Autodesk Inventor part; units mm, degrees
ref_plane "Piano di lavoro9" through (123.3139, -0.0528, 92.5382) normal (1, 0, 0) x (0, 0, -1)
ref_plane "Piano di lavoro11" through (123.3139, -0.0528, 92.5382) normal (1, 0, 0) x (0, 0, -1)
ref_plane "YZ Plane" through (0, 0, 0) normal (1, 0, 0) x (0, 1, 0)
ref_plane "Piano di lavoro9" through (123.3139, -0.0528, 92.5382) normal (1, 0, 0) x (0, 0, -1)
sketch "Schizzo5" plane through (123.3139, -0.0528, 92.5382) normal (1, 0, 0) x (0, 0, -1)
  line L0 (71.3231, 66.1847) -> (134.8231, 66.1847)
  line L1 (134.8231, 66.1847) -> (134.8231, 34.6847)
  line L2 (134.8231, 34.6847) -> (71.3231, 34.6847)
  line L3 (71.3231, 34.6847) -> (71.3231, 66.1847)
  line L4 (71.3231, 34.6847) -> (81.3231, 34.6847)
  line L5 (81.3231, 34.6847) -> (81.3231, 29.6847)
  line L6 (81.3231, 29.6847) -> (71.3231, 29.6847)
  line L7 (134.8231, 34.6847) -> (124.8231, 34.6847)
  line L8 (124.8231, 34.6847) -> (124.8231, 29.6847)
  line L9 (124.8231, 29.6847) -> (134.8231, 29.6847)
  line L10 (71.3231, 66.1847) -> (81.3231, 66.1847)
  line L11 (81.3231, 66.1847) -> (81.3231, 69.1847)
  line L12 (81.3231, 69.1847) -> (71.3231, 69.1847)
  line L13 (134.8231, 66.1847) -> (124.8231, 66.1847)
  line L14 (124.8231, 66.1847) -> (124.8231, 69.1847)
  line L15 (124.8231, 69.1847) -> (134.8231, 69.1847)
  line L16 (71.3231, 69.1847) -> (68.3231, 69.1847)
  line L17 (68.3231, 69.1847) -> (68.3231, 29.6847)
  line L18 (68.3231, 29.6847) -> (71.3231, 29.6847)
  line L19 (71.3231, 34.6847) -> (71.3231, 66.1847)
  line L20 (134.8231, 69.1847) -> (137.8231, 69.1847)
  line L21 (137.8231, 69.1847) -> (137.8231, 29.6847)
  line L22 (137.8231, 29.6847) -> (134.8231, 29.6847)
  point P0 (92.5382, 0.0528)
  dimension "d18" = 63.5
  dimension "d19" = 31.5
  dimension "d20" = 10
  dimension "d21" = 5
  dimension "d22" = 10
  dimension "d23" = 5
  dimension "d24" = 10
  dimension "d25" = 3
  dimension "d26" = 10
  dimension "d27" = 3
  dimension "d28" = 3
  dimension "d29" = 3
extrude "Estrusione3" add sketch "Schizzo5" against normal blind 100 contours L3 L2 L5 L6 L18 L17 L16 L12 L11 L0 | L14 L15 L20 L21 L22 L9 L8 L2 L1 L0
ref_plane "Piano di lavoro11" through (123.3139, -0.0528, 92.5382) normal (1, 0, 0) x (0, 0, -1)
sketch "Schizzo6" plane through (123.3139, -0.0528, 92.5382) normal (1, 0, 0) x (0, 0, -1)
  line L0 (71.3231, 66.1847) -> (81.3231, 66.1847)
  line L1 (81.3231, 34.6847) -> (71.3231, 34.6847)
  line L2 (81.3231, 29.6847) -> (81.3231, 34.6847)
  line L3 (134.8231, 66.1847) -> (134.8231, 34.6847)
  line L4 (71.3231, 34.6847) -> (71.3231, 66.1847)
  line L5 (68.3231, 99.6847) -> (137.155, 99.6847)
  line L6 (124.8231, 69.1847) -> (137.8231, 69.1847)
  line L7 (137.8231, 69.1847) -> (134.8231, 69.1847)
  line L8 (134.8231, 69.1847) -> (134.8231, 79.6847)
  line L9 (137.8231, 79.6847) -> (137.8231, 69.1847)
  line L10 (71.3231, 69.1847) -> (71.3231, 79.6847)
  line L11 (68.3231, 79.6847) -> (68.3231, 69.1847)
  line L12 (115.0731, 79.6847) -> (134.8231, 79.6847)
  line L13 (137.8231, 79.6847) -> (137.8231, 82.6847)
  line L14 (137.8231, 82.6847) -> (118.0731, 82.6847)
  line L15 (91.0731, 79.6847) -> (71.3231, 79.6847)
  line L16 (68.3231, 79.6847) -> (68.3231, 82.6847)
  line L17 (68.3231, 82.6847) -> (88.0731, 82.6847)
  line L18 (91.0731, 82.6847) -> (93.0731, 82.6847)
  line L19 (93.0731, 82.6847) -> (93.0731, 79.6847)
  line L20 (93.0731, 79.6847) -> (91.0731, 79.6847)
  line L21 (115.0731, 82.6847) -> (113.0731, 82.6847)
  line L22 (113.0731, 82.6847) -> (113.0731, 79.6847)
  line L23 (113.0731, 79.6847) -> (115.0731, 79.6847)
  line L24 (91.0731, 82.6847) -> (91.0731, 84.6847)
  line L25 (88.0731, 82.6847) -> (88.0731, 85.6847)
  line L26 (93.0731, 85.6847) -> (93.0731, 84.6847)
  line L27 (93.0731, 84.6847) -> (91.0731, 84.6847)
  line L28 (113.0731, 84.6847) -> (115.0731, 84.6847)
  line L29 (93.0731, 85.6847) -> (93.0731, 86.6847)
  line L30 (88.0731, 85.6847) -> (88.0731, 86.6847)
  line L31 (88.0731, 86.6847) -> (93.0731, 86.6847)
  line L32 (113.0731, 84.6847) -> (113.0731, 86.6847)
  line L33 (113.0731, 86.6847) -> (118.0731, 86.6847)
  line L34 (118.0731, 86.6847) -> (118.0731, 82.6847)
  line L35 (115.0731, 84.6847) -> (115.0731, 82.6847)
  line L36 (68.3231, 69.1847) -> (81.3231, 69.1847)
  line L37 (71.3231, 69.1847) -> (68.3231, 69.1847)
  point P0 (92.5382, 0.0528)
  point P1 (68.3231, 29.6847)
  dimension "d32" = 70
  dimension "d33" = 31.5
  dimension "d35" = 63.5
  dimension "d37" = 3
  dimension "d38" = 10.5
  dimension "d39" = 3
  dimension "d40" = 10.5
  dimension "d43" = 3
  dimension "d44" = 3
  dimension "d45" = 2
  dimension "d46" = 2
  dimension "d47" = 2
  dimension "d50" = 2
  dimension "d54" = 2
  dimension "d55" = 4
  dimension "d56" = 5
  dimension "d57" = 2
  dimension "d58" = 2
  dimension "d59" = 5
extrude "Estrusione4" add sketch "Schizzo6" against normal blind 50
sketch "Schizzo7" plane through (123.3139, 29.6319, -32.2849) normal (0, 0, 1) x (1, 0, 0)
  line L0 (0, 5) -> (0, 0)
  line L1 (0, 5) -> (-100, 5)
  line L2 (-100, 0) -> (-100, 5)
  line L3 (0, 0) -> (-100, 0)
  point P0 (-123.3139, -29.6319)
extrude "Estrusione5" add sketch "Schizzo7" along normal blind 47.25
sketch "Schizzo8" plane through (123.3139, -0.0528, 92.5382) normal (1, 0, 0) x (0, 0, -1)
  line L0 (71.3231, 66.1847) -> (71.3231, 34.6847)
  line L1 (71.3231, 34.6847) -> (65.0934, 34.6847)
  line L2 (134.8231, 34.6847) -> (141.848, 34.6847)
  line L3 (137.8231, 29.6847) -> (137.8231, 82.6847)
  line L4 (68.3231, 29.6847) -> (68.3231, 69.1847)
  line L5 (137.8231, 34.6847) -> (68.3231, 34.6847)
  line L6 (68.3231, 34.6847) -> (68.3231, 29.6797)
  line L7 (137.8231, 29.6797) -> (137.8231, 34.6847)
  line L8 (68.3231, 29.6847) -> (137.86, 29.6847)
  line L9 (93.0823, 34.6854) -> (113.0823, 34.6854)
  line L10 (113.0823, 34.6854) -> (113.0823, 29.6854)
  line L11 (113.0823, 29.6854) -> (93.0823, 29.6854)
  line L12 (93.0823, 29.6854) -> (93.0823, 34.6854)
  line L13 (113.0823, 34.6854) -> (93.0823, 34.6854)
  line L14 (93.0823, 34.6854) -> (93.0823, 29.6854)
  line L15 (93.0823, 29.6854) -> (113.0823, 29.6854)
  line L16 (113.0823, 29.6854) -> (113.0823, 34.6854)
  point P0 (92.5382, 0.0528)
  point P1 (103.0823, 32.1854)
  point P2 (103.0823, 32.1854)
  point P3 (113.0823, 34.6847)
  point P4 (93.0823, 34.6847)
  dimension "d82" = 20
  dimension "d83" = 5
extrude "Estrusione6" add sketch "Schizzo8" along normal blind 25 contours L5 L10 L8 L12
sketch "Schizzo9" plane through (23.3139, -0.0528, 92.5382) normal (-1, 0, 0) x (0, 0, 1)
  line L0 (-71.3231, 66.1847) -> (-71.3231, 34.6847)
  line L1 (-71.3231, 34.6847) -> (-67.9708, 34.6847)
  line L2 (-68.3231, 82.6847) -> (-68.3231, 29.6847)
  line L3 (-68.3231, 29.6847) -> (-137.8231, 29.6847)
  line L4 (-68.3231, 34.6847) -> (-137.8231, 34.6847)
  line L5 (-137.8231, 34.6847) -> (-137.8231, 29.6847)
  line L6 (-137.8231, 29.6847) -> (-68.3231, 29.6847)
  line L7 (-68.3231, 29.6847) -> (-68.3231, 34.6847)
  line L8 (-113.0731, 34.6847) -> (-93.0731, 34.6847)
  line L9 (-93.0731, 34.6847) -> (-93.0731, 29.6847)
  line L10 (-93.0731, 29.6847) -> (-113.0731, 29.6847)
  line L11 (-113.0731, 29.6847) -> (-113.0731, 34.6847)
  point P0 (-92.5382, 0.0528)
  point P1 (-103.0731, 32.1847)
  point P2 (-103.0731, 32.1847)
  dimension "d86" = 20
  dimension "d87" = 5
extrude "Estrusione7" add sketch "Schizzo9" along normal blind 25 contours L9 L3 L11 L4
sketch "Schizzo10" plane through (23.3139, 34.6319, 21.2151) normal (0, 1, 0) x (1, 0, 0)
  line L0 (-25, 21.75) -> (-25, 41.75)
  line L1 (-25, 31.75) -> (-20, 31.75)
  circle A0 centre (-20, 31.75) radius 0.5
  line L2 (125, 41.7592) -> (125, 21.7592)
  line L3 (125, 31.7592) -> (120, 31.7592)
  circle A1 centre (120, 31.7592) radius 0.5
  point P0 (-23.3139, 21.2151)
  dimension "d90" = 5
  dimension "d91" = 1
  dimension "d92" = 5
  dimension "d93" = 1
sketch "Schizzo11" plane through (148.3139, -0.0528, 92.5382) normal (1, 0, 0) x (0, 0, -1)
  line L0 (113.0823, 34.6847) -> (93.0823, 34.6847)
  line L1 (113.0823, 29.6854) -> (113.0823, 34.6847)
  line L2 (93.0823, 34.6847) -> (113.0823, 34.6847)
  line L3 (113.0823, 34.6847) -> (113.0823, 29.6854)
  line L4 (113.0823, 29.6854) -> (93.0823, 29.6854)
  line L5 (93.0823, 29.6854) -> (93.0823, 34.6847)
  point P0 (92.5382, 0.0528)
extrude "Estrusione8" add sketch "Schizzo11" along normal blind 5
sketch "Schizzo12" plane through (-1.6861, -0.0528, 92.5382) normal (-1, 0, 0) x (0, 0, 1)
  line L0 (-113.0731, 34.6847) -> (-134.8231, 34.6847)
  line L1 (-113.0823, 29.6854) -> (-93.0823, 29.6854)
  line L2 (-113.0731, 34.6847) -> (-93.0823, 34.6847)
  line L3 (-93.0823, 34.6847) -> (-93.0823, 29.6854)
  line L4 (-93.0823, 29.6854) -> (-113.0731, 29.6854)
  line L5 (-113.0731, 29.6854) -> (-113.0731, 34.6847)
  point P0 (-92.5382, 0.0528)
extrude "Estrusione9" add sketch "Schizzo12" along normal blind 5
sketch "Schizzo14" plane through (153.3139, -0.0528, 92.5382) normal (1, 0, 0) x (0, 0, -1)
  line L0 (93.0823, 34.6847) -> (71.3231, 34.6847)
  line L1 (68.3231, 29.6847) -> (137.8231, 29.6847)
  line L2 (93.0823, 34.6847) -> (113.0814, 34.6847)
  line L3 (113.0814, 34.6847) -> (113.0814, 29.6847)
  line L4 (113.0814, 29.6847) -> (93.0823, 29.6847)
  line L5 (93.0823, 29.6847) -> (93.0823, 34.6847)
  point P0 (92.5382, 0.0528)
extrude "Estrusione10" add sketch "Schizzo14" along normal blind 7.5
sketch "Schizzo15" plane through (-6.6861, -0.0528, 92.5382) normal (-1, 0, 0) x (0, 0, 1)
  line L0 (-93.0823, 29.6854) -> (-113.0814, 29.6854)
  line L1 (-113.0814, 34.6847) -> (-93.0823, 34.6847)
  line L2 (-93.0823, 29.6854) -> (-113.0814, 29.6854)
  line L3 (-113.0814, 29.6854) -> (-113.0814, 34.6847)
  line L4 (-113.0814, 34.6847) -> (-93.0823, 34.6847)
  line L5 (-93.0823, 34.6847) -> (-93.0823, 29.6854)
  point P0 (-92.5382, 0.0528)
extrude "Estrusione11" add sketch "Schizzo15" along normal blind 7.5
properties part number "pignat_2_Stampa 3D"
Could you check a few things on this model? Use its own coordinates, in mm. A direction names the side the tool comes from. Round coordinates to 2 decimals unless told otherwise and drop trailing zeros. Loops run counter-clockwise (first coordinate to the right, second up) from the corner with the lowest first, then second, coordinate; pieces in that order, holes last. Notation, with made-up numbers: (-21.75, -35) - (35.25, -35) arc R20 ccw to (35.25, -1) - close; hole circle Ø9 at (-3, -36). An arc over 180 degrees is marked (long way). Write item = value, one per line.
1) I'm going to push flat-ended pins straight in: P1, Ø3, axis at x = 86.5, y = 85.5, coming from the -Z side; P2, Ø4, axis at x = 62, z = 20.5, coming from the +Y side; P3, Ø10, axis at y = 43, z = -34, coming from the -X side; P4, Ø21.5, axis at x = 98.5, z = 15.5, coming from the +Y side. Where does each tip first touch, or does it pass through?
Computed:
P1 = -25.53
P2 = 69.13
P3 = through
P4 = 82.63
2) Imagine slicing it at A-A (y = 54.5). Please give me the cut outline in (x, z).
Computed:
outline = (23.31, -45.28) - (123.31, -45.28) - (123.31, -42.28) - (23.31, -42.28) - close; (23.31, 21.22) - (123.31, 21.22) - (123.31, 24.22) - (23.31, 24.22) - close
3) On a 3-axis mill with a long thin cutter (end or side, diameter ignored), from which of +Z, -Z, +X, -X, +Y, -Y can I reach the whole of each face in a straight line? I mean faces 4 (the flat face through (23.314, 43, 22)), 5 (the flat face through (123.314, 56, 22)), 6 (the flat face through (74, 50, 21.215)). Say none if no direction works.
Computed:
face_4 = +Z, -X, +Y, -Y
face_5 = +Z, +X, +Y, -Y
face_6 = +X, -X
4) I need wall thicknesses on line 1 along Y through (x, z) = (102, 13.5); line 2 along Y through (x, z) = (33.5, -41); line 3 along Z through (x, y) = (104, 56). Which ranges of each line are inside material? Lowest first, please. Write a range as from..to.
Computed:
line_1 = 29.63..34.63, 66.13..69.13, 79.63..82.63
line_2 = 29.63..34.63, 66.13..69.13
line_3 = -45.28..-42.28, 21.22..24.22
5) Imagine slicing it at B-B (z = 14). Please give me the cut outline in (x, y).
Computed:
outline = (23.31, 29.63) - (123.31, 29.63) - (123.31, 34.63) - (23.31, 34.63) - close; (23.31, 66.13) - (123.31, 66.13) - (123.31, 69.13) - (23.31, 69.13) - close; (73.31, 79.63) - (123.31, 79.63) - (123.31, 82.63) - (73.31, 82.63) - close
6) If we mould it in two halves opening along Z, with no side actions, what happens to faces 1 (the flat face through (99, 74, 21.215)), 2 (the flat face through (99, 82.632, -36)), 3 (the flat face through (11, 32, -0.535))? For each: pulls with the +Z half, pulls with the -Z half, needs draft (parallel to the pull), parting line crosses it, or undercut.
Computed:
face_1 = undercut
face_2 = needs draft
face_3 = pulls with the +Z half
7) Imagine slicing it at C-C (x = 48.5). Please give me the cut outline in (y, z).
Computed:
outline = (29.63, -45.28) - (69.13, -45.28) - (69.13, -32.28) - (66.13, -32.28) - (66.13, -42.28) - (34.63, -42.28) - (34.63, 21.22) - (66.13, 21.22) - (66.13, 11.22) - (69.13, 11.22) - (69.13, 24.22) - (29.63, 24.22) - close
